Check sheet for the drawn part. Datum: minimum x, y, z corner. Units: mm. A direction names the side the tool comes from. Give positions to 0.01 mm unless a question says otherwise; leave off trailing zeros. Write each loop counter-clockwise with the first axis right and the second up, starting at its lowest first coordinate (ties: lowest second). Pieces come first, ordered by that corner, then holes. Notation, with made-up numbers: (41, 74.5) -> (99, 74.5) arc R34 cw to (99, 110.5) -> close; hole circle Ø11 at (60, 77). An arc over 180 degrees is marked (long way). Answer as CSV lines item,"result". Start each with the question number.
1) Gauge pin test, flat ends, axial feed: pin 1 Ø4.5 at (x, y) = (52.5, 8.5) entering from +Z; pin 2 Ø1.5 at (x, y) = (21.5, 2) entering from +Z; pin 3 Ø1.5 at (x, y) = (52.5, 5.5) entering from +Z. Record the tip position at first contact, or that the pin passes through.
2) Material ranges on L1, parallel to Y at x = 31, z = 68.25; L2, parallel to X at y = 5, z = 35; L3, parallel to X at y = 4.75, z = 14, recorded low to high.
3) Mould release check, pull along X, two halves, no side actions. Record for the marked faces 4, 5 and 6: released by +X, released by -X, zero draft, split by the parting line, or undercut.
4) Sectioned sample at A-A on y = 6. Record the cut outline in (x, z), and give its area (3 significant figures).
5) Tool access check on the marked faces 1, 2 and 3. Record the directions out of +Z, -Z, +X, -X, +Y, -Y that give a thin tool (end or side, any length) a straight path to the whole face; none if there is none.
6) Sectioned sample at C-C on x = 33.5. Record the cut outline in (y, z), and give its area (3 significant figures).
7) Sectioned sample at B-B on z = 57. Record the cut outline in (x, y), and give its area (3 significant figures).
8) Sectioned sample at D-D on z = 19. Record the cut outline in (x, y), and give its area (3 significant figures).
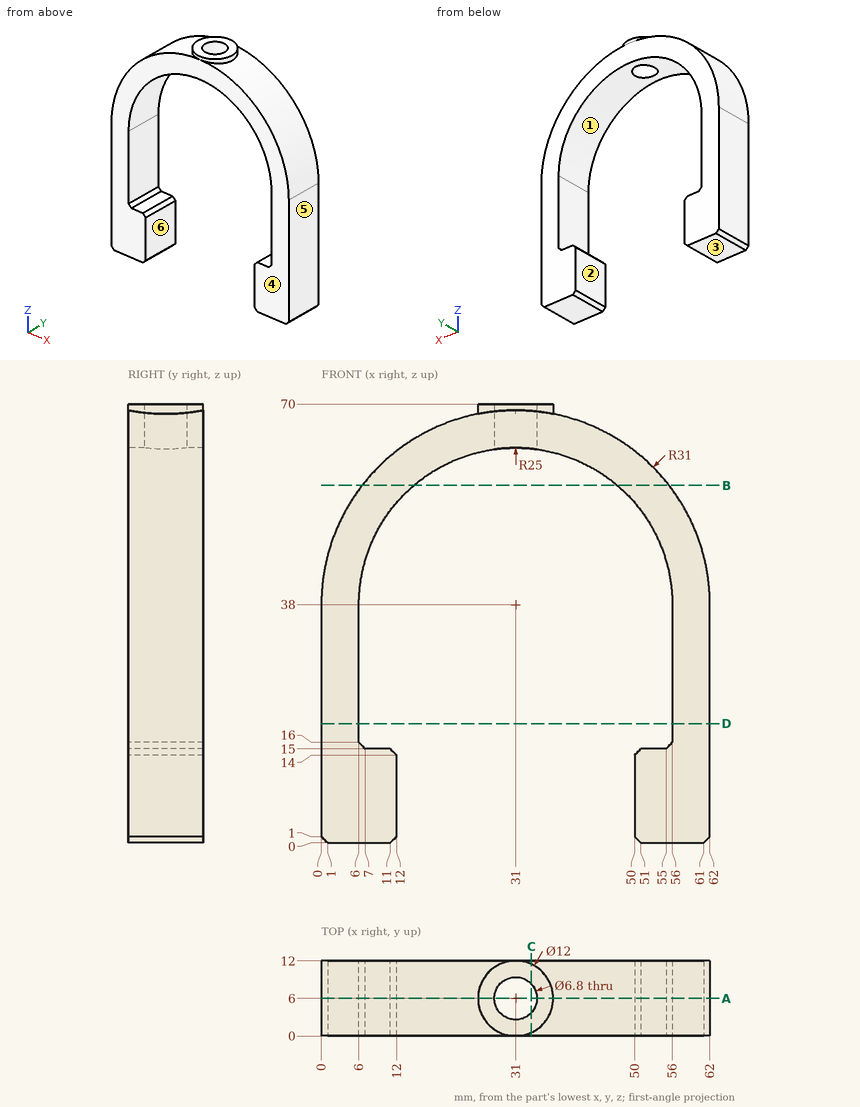
Ans:
1,pin 1,"stops at z = 62.3"
1,pin 2,"stops at z = 67.74"
1,pin 3,"stops at z = 61.03"
2,L1,"y = 0 to 2.6, 9.4 to 12"
2,L2,"x = 0 to 6, 56 to 62"
2,L3,"x = 0 to 12, 50 to 62"
3,face 4,"zero draft"
3,face 5,"released by +X"
3,face 6,"undercut"
4,outline,"(0, 1) -> (1, 0) -> (11, 0) -> (12, 1) -> (12, 14) -> (11, 15) -> (7, 15) -> (6, 16) -> (6, 38) arc R25 cw to (27.6, 62.77) -> (27.6, 70) -> (25, 70) -> (25, 68.41) arc R31 ccw to (0, 38) -> close; (34.4, 62.77) arc R25 cw to (56, 38) -> (56, 16) -> (55, 15) -> (51, 15) -> (50, 14) -> (50, 1) -> (51, 0) -> (61, 0) -> (62, 1) -> (62, 38) arc R31 ccw to (37, 68.41) -> (37, 70) -> (34.4, 70) -> close"
4,area,"1,130 mm²"
5,face 1,"+Y, -Y"
5,face 2,"-Z, +Y, -Y"
5,face 3,"-Z, +X, -X, +Y, -Y"
6,outline,"(0, 62.87) -> (3.7, 62.87) -> (3.7, 70) -> (0.55, 70) -> (0.55, 68.9) -> (0, 68.9) -> close; (8.3, 62.87) -> (12, 62.87) -> (12, 68.9) -> (11.45, 68.9) -> (11.45, 70) -> (8.3, 70) -> close"
6,area,"51.5 mm²"
7,outline,"(6.51, 0) -> (14.75, 0) -> (14.75, 12) -> (6.51, 12) -> close; (47.25, 0) -> (55.49, 0) -> (55.49, 12) -> (47.25, 12) -> close"
7,area,"198 mm²"
8,outline,"(0, 0) -> (6, 0) -> (6, 12) -> (0, 12) -> close; (56, 0) -> (62, 0) -> (62, 12) -> (56, 12) -> close"
8,area,"144 mm²"
